from build123d import *

# Parameters (mm, degrees)
SKETCH1_R                  = 11.1125
EXTRUDE1_DEPTH             = 12.7
BUSHING_SIDE_FILLETS_R     = 0.79375
MOUNT_SIDE_FILLETS_R       = 0.79375
F_1_4_MOUNTING_HOLES_D     = 5.1054
F_1_4_MOUNTING_HOLES_DEPTH = 19.05
F_1_4_MOUNTING_HOLES_TIP   = 1.533816902
CUT_EXTRUDE1_DEPTH         = 51.649420448
FILLET1_R                  = 2.5


with BuildPart() as part:
    # Sketch1 → Extrude1 (new, symmetric)
    with BuildSketch(Plane(origin=(0, 0, 0), x_dir=(1, 0, 0), z_dir=(0, 0, -1))):
        with BuildLine():
            Line((0.5, 12.690153663), (0.5, 30.5587))
            Line((0.5, 30.5587), (1.5, 30.5587))
            Line((1.5, 30.5587), (1.5, 14.623269128))
            ThreePointArc((1.5, 14.623269128), (10.911920088, 9.849873096), (14.7, 0))
            Line((14.7, 0), (17.705953405, 0))
            Line((17.705953405, 0), (17.705953405, 40.0837))
            Line((17.705953405, 40.0837), (-17.705953405, 40.0837))
            Line((-17.705953405, 40.0837), (-17.705953405, 0))
            Line((-17.705953405, 0), (-14.7, 0))
            ThreePointArc((-14.7, 0), (-10.911920088, 9.849873096), (-1.5, 14.623269128))
            Line((-1.5, 14.623269128), (-1.5, 30.5587))
            Line((-1.5, 30.5587), (-0.5, 30.5587))
            Line((-0.5, 30.5587), (-0.5, 12.690153663))
            ThreePointArc((-0.5, 12.690153663), (0, -12.7), (0.5, 12.690153663))
        make_face()
        Circle(SKETCH1_R, mode=Mode.SUBTRACT)
    extrude(amount=EXTRUDE1_DEPTH, both=True)

    # Bushing-side fillets
    bushing_side_fillets_edges = [part.edges().sort_by_distance(p)[0] for p in [
        (-0.5, -12.690153663, 0),
        (0.5, -12.690153663, 0),
    ]]
    fillet(bushing_side_fillets_edges, radius=BUSHING_SIDE_FILLETS_R)

    # Mount-side fillets
    mount_side_fillets_edges = [part.edges().sort_by_distance(p)[0] for p in [
        (-0.5, -30.5587, 0),
        (0.5, -30.5587, 0),
    ]]
    fillet(mount_side_fillets_edges, radius=MOUNT_SIDE_FILLETS_R)

    # 1/4 Mounting holes
    with Locations(Plane.XZ.offset(40.0837)):
        with Locations((-12.7, 0), (12.7, 0)):
            Hole(F_1_4_MOUNTING_HOLES_D / 2, depth=F_1_4_MOUNTING_HOLES_DEPTH)
            with Locations((0, 0, -(F_1_4_MOUNTING_HOLES_DEPTH + F_1_4_MOUNTING_HOLES_TIP / 2))):  # 118° drill point
                Cone(0, F_1_4_MOUNTING_HOLES_D / 2, F_1_4_MOUNTING_HOLES_TIP, mode=Mode.SUBTRACT)

    # Sketch6 → Cut-Extrude1 (cut, through all)
    with BuildSketch(Plane(origin=(0, 0, -12.7), x_dir=(-1, 0, 0), z_dir=(0, 0, -1))):
        with BuildLine():
            Line((0.5, -29.6587), (0.5, -36.4087))
            ThreePointArc((0.5, -36.4087), (1, -36.9087), (1.5, -36.4087))
            Line((1.5, -36.4087), (1.5, -30.5587))
            Line((1.5, -30.5587), (1.4, -30.5587))
            ThreePointArc((1.4, -30.5587), (0.763603897, -30.295096103), (0.5, -29.6587))
        make_face()
        with BuildLine():
            Line((-1.5, -30.5587), (-1.4, -30.5587))
            ThreePointArc((-1.4, -30.5587), (-0.763603897, -30.295096103), (-0.5, -29.6587))
            Line((-0.5, -29.6587), (-0.5, -36.4087))
            ThreePointArc((-0.5, -36.4087), (-1, -36.9087), (-1.5, -36.4087))
            Line((-1.5, -36.4087), (-1.5, -30.5587))
        make_face()
    extrude(amount=-CUT_EXTRUDE1_DEPTH, mode=Mode.SUBTRACT)

    # Fillet1
    fillet1_edges = [part.edges().sort_by_distance(p)[0] for p in [
        (-14.7, 0, 0),
        (-1.5, -14.623269128, 0),
        (1.5, -14.623269128, 0),
        (14.7, 0, 0),
    ]]
    fillet(fillet1_edges, radius=FILLET1_R)


solid = part.part
Could you check a few things on this model? Use its own coordinates, in mm. A direction names the side the tool comes from. Round coordinates to 2 decimals unless told otherwise and drop trailing zeros. Order: outer loops, then holes, each group sorted by start corner. A loop starts at its lowest first (then second) coordinate and runs counter-clockwise, first axis right, second up. Notation, with made-up numbers: M -22,18 L -11,18 A27 ccw -11,45 Z; hole C -22.75,-38.75 d1. An arc over 180 degrees is marked long. One line per item, written item: value.
(1) Imagine slicing it at B-B (y = -1). Write out the boundary of the cut face in (x, z).
Ans:
outline: M -17.71,-12.7 L -15.02,-12.7 L -15.02,12.7 L -17.71,12.7 Z; M -12.66,-12.7 L -11.07,-12.7 L -11.07,12.7 L -12.66,12.7 Z; M 11.07,-12.7 L 12.66,-12.7 L 12.66,12.7 L 11.07,12.7 Z; M 15.02,-12.7 L 17.71,-12.7 L 17.71,12.7 L 15.02,12.7 Z
(2) Imagine slicing it at D-D (y = -12). Write out the boundary of the cut face in (x, z).
Ans:
outline: M -17.71,-12.7 L -8.49,-12.7 L -8.49,12.7 L -17.71,12.7 Z; M -4.16,-12.7 L 4.16,-12.7 L 4.16,12.7 L -4.16,12.7 Z; M 8.49,-12.7 L 17.71,-12.7 L 17.71,12.7 L 8.49,12.7 Z
(3) Which directions (+Z, -Z, +X, -X, +Y, -Y) give clear straight access to the entire face, cutting with the end or side of a thin tool? Please do faces 4 (the flat face through (0, -40.084, 0)), 5 (the cylindrical face through (15.402, -0.592, -0.178)), 6 (the flat face through (-0.5, -25, 0)).
Ans:
face 4: +Z, -Z, +X, -X, -Y
face 5: +Z, -Z, +Y
face 6: +Z, -Z
(4) If we mould it in two halves opening along Z, with no side actions, what happens to faces 1 (the conical face through (12.3, -19.8, -0.3)), 2 (the cylindrical face through (-0.54, 12.69, -0.18)), 3 (the flat face through (0, -20, -12.7))? For each: released by +Z, released by -Z, zero draft, split by the parting line, or undercut.
Ans:
face 1: undercut
face 2: zero draft
face 3: released by -Z
(5) I need wall thicknesses on line 1 along X through (y, z) = (-36, 4.25); line 2 along X through (y, z) = (-31, 0); line 3 along Y through (x, z) = (-8, -10). Which ranges of each line are inside material? Lowest first, please. Write a range as from..to.
Ans:
line 1: x = -17.71..-1.5, -0.5..0.5, 1.5..17.71
line 2: x = -17.71..-15.25, -10.15..-1.5, -0.5..0.5, 1.5..10.15, 15.25..17.71
line 3: y = -40.08..-12.33, -9.86..-7.71, 7.71..9.86
(6) Imagine slicing it at C-C (x = -8). Write out the boundary of the cut face in (y, z), and give its area (3 significant figures).
Ans:
outline: M -40.08,-12.7 L -12.33,-12.7 L -12.33,12.7 L -40.08,12.7 Z; M -9.86,-12.7 L -7.71,-12.7 L -7.71,12.7 L -9.86,12.7 Z; M 7.71,-12.7 L 9.86,-12.7 L 9.86,12.7 L 7.71,12.7 Z
area: 814 mm^2
(7) Imagine slicing it at A-A (z = -8.25). Write out the boundary of the cut face in (x, y) (1 decimal).
Ans:
outline: M -17.7,-40.1 L 17.7,-40.1 L 17.7,0 L 17,0 A2.5 ccw 14.5,-2.1 A14.7 cw 3.4,-14.3 A2.5 ccw 1.5,-16.7 L 1.5,-36.4 A0.5 cw 0.5,-36.4 L 0.5,-13.4 A0.8 cw 1.2,-12.6 A12.7 ccw long -1.2,-12.6 A0.8 cw -0.5,-13.4 L -0.5,-36.4 A0.5 cw -1.5,-36.4 L -1.5,-16.7 A2.5 ccw -3.4,-14.3 A14.7 cw -14.5,-2.1 A2.5 ccw -17,0 L -17.7,0 Z; hole C 0,0 d22.2
(8) I'm going to push flat-ended pins straight in: P1, Ø0.8, axis at x = 17.5, z = 6.5, coming from the +Y side; P2, Ø8, axis at x = 12.7, z = 0, coming from the +Y side; P3, Ø4.5, axis at x = -12.7, z = 0, coming from the -Y side. Where does each tip first touch, or does it pass through?
Ans:
P1: stops at y = 0
P2: stops at y = 9.25
P3: stops at y = -20.85
